Input: part model. Units: mm. Frame: model coordinates. A direction names the side the tool comes from. Round coordinates to 2 decimals unless told otherwise and drop trailing zeros. Loops run counter-clockwise (first coordinate to the right, second up) from the corner with the lowest first, then second, coordinate; pieces in that order, holes last. Notation, with made-up numbers: (22.25, -33.75) -> (32.25, -33.75) arc R14 cw to (32.25, -6.75) -> close; hole circle Ø2 at (18, 11.25). An arc over 180 degrees is marked (long way). Answer as a JSON object with one key per item and string values.
```python
from build123d import *

# Parameters (mm, degrees)
SKETCH1_W           = 58.42
SKETCH1_H           = 58.42
BOSS_EXTRUDE1_DEPTH = 56
SKETCH2_R           = 30
BOSS_EXTRUDE2_DEPTH = 72
SKETCH3_R           = 6
BOSS_EXTRUDE3_DEPTH = 30
SKETCH4_R           = 2.5
CUT_EXTRUDE1_DEPTH  = 25.4
SKETCH5_W           = 2.5
SKETCH5_H           = 4
CUT_EXTRUDE2_DEPTH  = 20


with BuildPart() as part:
    # Sketch1 → Boss-Extrude1 (new body)
    with BuildSketch(Plane(origin=(0, 0, 0), x_dir=(1, 0, 0), z_dir=(0, 1, 0))):
        Rectangle(SKETCH1_W, SKETCH1_H)
    extrude(amount=BOSS_EXTRUDE1_DEPTH)

    # Sketch2 → Boss-Extrude2 (add)
    with BuildSketch(Plane(origin=(0, 56, 0), x_dir=(1, 0, 0), z_dir=(0, 1, 0))):
        Circle(SKETCH2_R)
    extrude(amount=BOSS_EXTRUDE2_DEPTH)

    # Sketch3 → Boss-Extrude3 (add)
    with BuildSketch(Plane(origin=(0, 128, 0), x_dir=(1, 0, 0), z_dir=(0, 1, 0))):
        Circle(SKETCH3_R)
    extrude(amount=BOSS_EXTRUDE3_DEPTH)

    # Sketch4 → Cut-Extrude1 (cut)
    with BuildSketch(Plane(origin=(0, 128, 0), x_dir=(1, 0, 0), z_dir=(0, 1, 0))):
        with Locations((-13.611805538, 13.611805538)):
            Circle(SKETCH4_R)
        with Locations((13.611805538, 13.611805538)):
            Circle(SKETCH4_R)
        with Locations((13.611805538, -13.611805538)):
            Circle(SKETCH4_R)
        with Locations((-13.611805538, -13.611805538)):
            Circle(SKETCH4_R)
    extrude(amount=-CUT_EXTRUDE1_DEPTH, mode=Mode.SUBTRACT)

    # Sketch5 → Cut-Extrude2 (cut)
    with BuildSketch(Plane(origin=(0, 158, 0), x_dir=(1, 0, 0), z_dir=(0, 1, 0))):
        with Locations((4.75, 0)):
            Rectangle(SKETCH5_W, SKETCH5_H)
    extrude(amount=-CUT_EXTRUDE2_DEPTH, mode=Mode.SUBTRACT)


solid = part.part
```
1) Section B-B, the plane z = 0. Output: boundary loops of the cut face in (x, y), plus the area to 3 significant figures.
Output:
{"outline": "(-30, 56) -> (-29.21, 56) -> (-29.21, 0) -> (29.21, 0) -> (29.21, 56) -> (30, 56) -> (30, 128) -> (6, 128) -> (6, 138) -> (3.5, 138) -> (3.5, 158) -> (-6, 158) -> (-6, 128) -> (-30, 128) -> close", "area": "7,900 mm^2"}
2) Section C-C, the plane y = 98.5. Output: boundary loops of the cut face in (x, z), plus the area to 3 significant figures.
Output:
{"outline": "circle Ø60 at (0, 0)", "area": "2,830 mm^2"}
3) Section D-D, the plane x = -14.5. Output: boundary loops of the cut face in (y, z).
Output:
{"outline": "(0, -29.21) -> (56, -29.21) -> (56, -26.26) -> (128, -26.26) -> (128, -15.95) -> (102.6, -15.95) -> (102.6, -11.27) -> (128, -11.27) -> (128, 11.27) -> (102.6, 11.27) -> (102.6, 15.95) -> (128, 15.95) -> (128, 26.26) -> (56, 26.26) -> (56, 29.21) -> (0, 29.21) -> close"}
4) Draft query along Z for faces 4 (the face through (14, 102.6, 14)), 5 (the face through (14, 102.6, -14)), 6 (the face through (29.21, 28, 0)), 7 (the face through (-4.76, 142.79, 3.65)). Return one class per face: +Z half, -Z half, draft (parallel to the pull), parting line (faces both ways), or undercut.
Output:
{"face 4": "undercut", "face 5": "undercut", "face 6": "draft", "face 7": "parting line"}
5) Contact query for flat-ended pins moving along their axis: P1, Ø2.5, axis at x = 13.5, z = 12.5, coming from the +Y side; P2, Ø8, axis at x = 7, y = 118, coming from the +Z side; P3, Ø1.5, axis at y = 87.5, z = -22.5, coming from the +X side. Output: stop coordinate, or through.
Output:
{"P1": "stops at y = 102.6", "P2": "stops at z = 29.85", "P3": "stops at x = 20.66"}
6) Section A-A, the plane x = -1. Output: boundary loops of the cut face in (y, z), plus the area to 3 significant figures.
Output:
{"outline": "(0, -29.21) -> (56, -29.21) -> (56, -29.98) -> (128, -29.98) -> (128, -5.92) -> (158, -5.92) -> (158, 5.92) -> (128, 5.92) -> (128, 29.98) -> (56, 29.98) -> (56, 29.21) -> (0, 29.21) -> close", "area": "7,940 mm^2"}
7) Reachability of faces 1 (the face through (-24, 56, -24)), 2 (the face through (-29.21, 28, 0)), 3 (the face through (-29.97, 91.5, -1.32)) from +Z, -Z, +X, -X, +Y, -Y: full face, straight path, thin tool, end or side. Return the list, or none.
Output:
{"face 1": "-Z, -X, +Y", "face 2": "+Z, -Z, -X, -Y", "face 3": "+Y"}
8) Ray query, probe 1 along Z at (x, y) = (7, 9); probe 2 along Y at (x, z) = (26.5, 10); probe 3 along Y at (x, z) = (17, -26). Return the intervals inside material, ascending.
Output:
{"probe 1": "z = -29.21 to 29.21", "probe 2": "y = 0 to 128", "probe 3": "y = 0 to 56"}
